Part model, mm, in its own coordinate system. Round coordinates to 2 decimals unless told otherwise and drop trailing zeros. Loops run counter-clockwise (first coordinate to the right, second up) from the corner with the lowest first, then second, coordinate; pieces in that order, holes last.
Autodesk Fusion 360 part; units mm, degrees
sketch "Sketch1" plane through (0, 0, 0) normal (0, 0, 1) x (-1, 0, 0)
  line L0 (-80, 0) -> (80, 0) construction
  line L1 (-71, -12.5) -> (-10, -12.5)
  line L2 (-10, -12.5) -> (-10, 12.5)
  line L3 (-10, 12.5) -> (-71, 12.5)
  line L4 (-71, 12.5) -> (-71, -12.5)
  line L5 (-71, -36.8646) -> (-71, 36.8646)
  line L6 (0, -80) -> (0, 80) construction
  line L7 (10, -12.5) -> (10, 12.5)
  line L8 (10, 12.5) -> (71, 12.5)
  line L9 (71, -12.5) -> (10, -12.5)
  line L10 (71, 12.5) -> (71, -12.5)
  line L11 (71, -36.8646) -> (71, 36.8646)
  arc A0 (71, 36.8646) -> (-71, 36.8646) centre (0, 0) ccw
  arc A1 (-71, -36.8646) -> (71, -36.8646) centre (0, 0) ccw
  dimension "d6" = 160
  dimension "d7" = 61
  dimension "d8" = 25
  dimension "d9" = 10
  dimension "d10" = 71
extrude "Extrude3" add sketch "Sketch1" along normal blind 5
sketch "Sketch3" plane through (0, 0, 5) normal (0, 0, 1) x (-1, 0, 0)
  line L0 (-71, 36.8646) -> (-71, 12.5)
  line L1 (-71, 12.5) -> (-10, 12.5)
  line L2 (-10, 12.5) -> (-10, -12.5)
  line L3 (-10, -12.5) -> (-71, -12.5)
  line L4 (-71, -12.5) -> (-71, -36.8646)
  arc A0 (-71, -36.8646) -> (71, -36.8646) centre (0, 0) ccw
  line L5 (71, -36.8646) -> (71, -12.5)
  line L6 (71, -12.5) -> (10, -12.5)
  line L7 (10, -12.5) -> (10, 12.5)
  line L8 (10, 12.5) -> (71, 12.5)
  line L9 (71, 12.5) -> (71, 36.8646)
  arc A1 (71, 36.8646) -> (-71, 36.8646) centre (0, 0) ccw
  line L10 (-70, 0) -> (70, 0) construction
  line L11 (0, 80) -> (0, -80) construction
  line L12 (21.5, -21.5) -> (-21.5, -21.5)
  line L13 (-21.5, -21.5) -> (-21.5, 21.5)
  line L14 (-21.5, 21.5) -> (21.5, 21.5)
  line L15 (21.5, 21.5) -> (21.5, -21.5)
  point P0 (-60.0095, 36.8646)
  point P1 (-34.3452, 61.4862)
  point P2 (0.0774, 70.4282)
  point P3 (34.4802, 61.4105)
  point P4 (60.0904, 36.7327)
  point P5 (-60.0095, -36.8646)
  point P6 (-34.3452, -61.4862)
  point P7 (0.0774, -70.4282)
  point P8 (34.4802, -61.4105)
  point P9 (60.0904, -36.7327)
  point P10 (21.5, -21.5)
  point P11 (-21.5, -21.5)
  point P12 (21.5, 21.5)
  point P13 (-21.5, 21.5)
  dimension "d20" = -117
  dimension "d25" = 43
  dimension "d26" = 43
hole "Hole2" at (-60.0904, 36.7327, 5) at (-34.4802, 61.4105, 5) at (-0.0774, 70.4282, 5) at (34.3452, 61.4862, 5) at (60.0095, 36.8646, 5) at (-60.0904, -36.7327, 5) at (-34.4802, -61.4105, 5) at (-0.0774, -70.4282, 5) at (34.3452, -61.4862, 5) at (60.0095, -36.8646, 5) direction (0, 0, -1) diameter 3.2 end through all
hole "Hole3" at (-21.5, 21.5, 5) at (21.5, 21.5, 5) at (-21.5, -21.5, 5) at (21.5, -21.5, 5) direction (0, 0, -1) diameter 2.7 end through all
equation "chasis_diameter = 160 mm"
equation "main_layer_thickness = 30 mm"
equation "motor_L = 21 mm"
equation "total_motor_body_length = 61 mm"
equation "standoff_height = 50 mm"
equation "d6 = chasis_diameter"
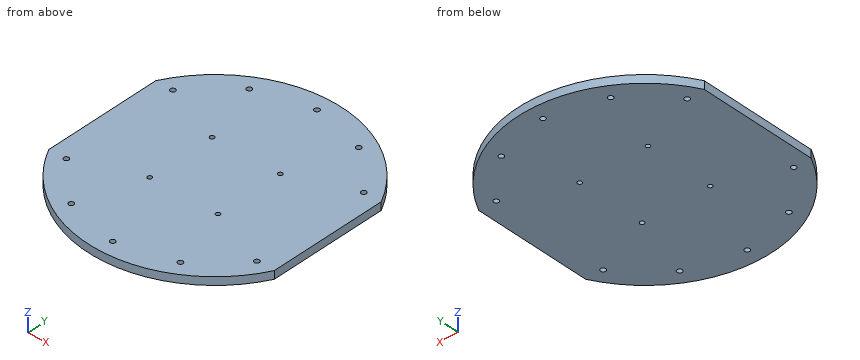
1) Slice it at A-A, the plane z = 1.45. Give the number of separate pieces and of enclosed holes in the cut face, then the cut area to 3 significant figures.
Values:
separate pieces: 1
enclosed holes: 14
area: 19,100 mm2
2) Slice it at B-B, the plane x = 39.5. Give the cut face in (y, z), then the cut area to 3 significant figures.
Values:
outline: (-69.57, 0) - (69.57, 0) - (69.57, 5) - (-69.57, 5) - close
area: 696 mm2
3) Slice it at C-C, the plane y = 51. Give the cut face in (x, z), then the cut area to 3 significant figures.
Values:
outline: (-61.64, 0) - (61.64, 0) - (61.64, 5) - (-61.64, 5) - close
area: 616 mm2
4) Wall check: line 1 along X through (y, z) = (21.5, 3.15); line 2 along Y through (x, z) = (-21, 2.2); line 3 along X through (y, z) = (35.5, 0.95). Give the ranges that are in metal, low to high.
Values:
line 1: x = -71 to -22.85, -20.15 to 20.15, 22.85 to 71
line 2: y = -77.19 to -22.75, -20.25 to 20.25, 22.75 to 77.19
line 3: x = -71 to -61.11, -59.07 to 59.17, 60.84 to 71
5) Drop flat-ended pins along their axis: pin 1 Ø2 at (x, y) = (-21.5, -21.5) entering from -Z (1 decimal); pin 2 Ø2 at (y, z) = (-53, 0.5) entering from +X; pin 3 Ø3 at (x, z) = (48, 2) entering from +Y. Give the stop position or say it passes through.
Values:
pin 1: passes through
pin 2: stops at x = 60.79
pin 3: stops at y = 65.1
